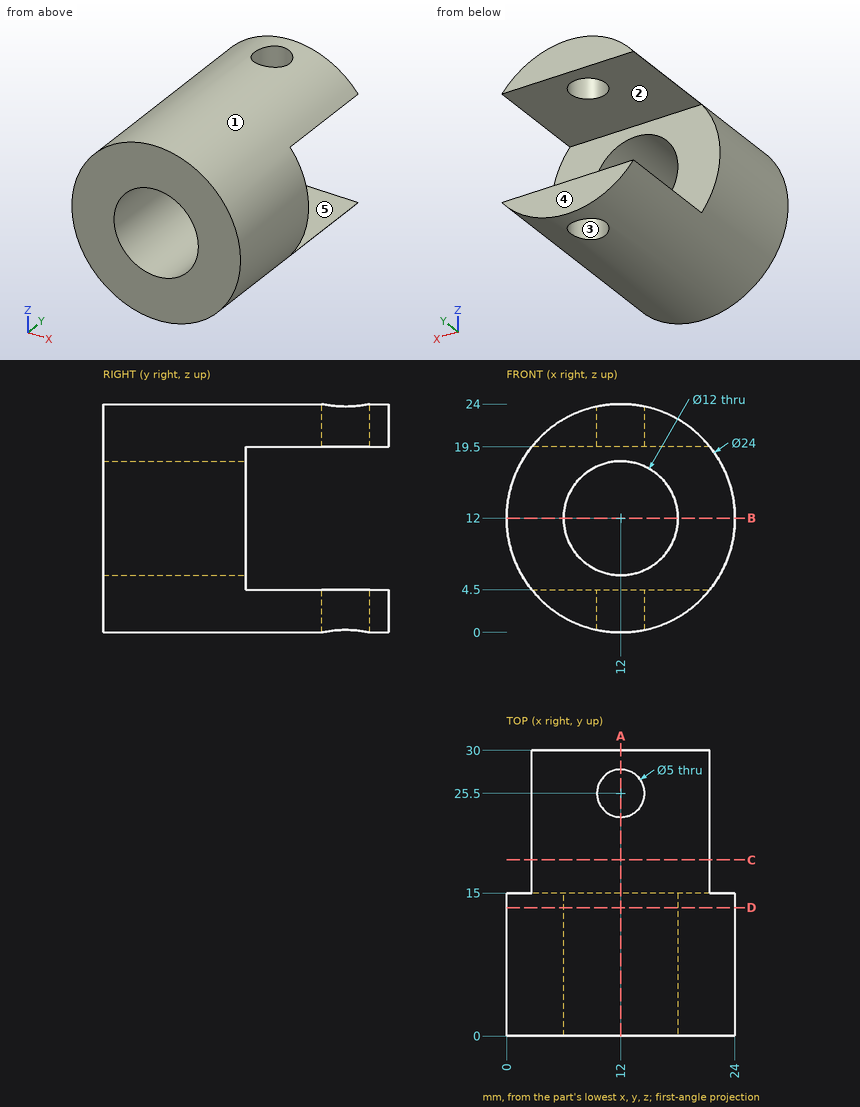
Verification items for this drawing (mm, ordinates from the low corner). A direction names the side the tool comes from. Round coordinates to 2 decimals unless told otherwise and drop trailing zeros. Write each loop counter-clockwise with the first axis right and the second up, starting at its lowest first coordinate (ties: lowest second). Pieces come first, ordered by that corner, then holes. Notation, with made-up numbers: (84, 89.5) - (118, 89.5) arc R25 ccw to (118, 116.5) - close; hole circle Ø6 at (-20, 75). An arc over 180 degrees is marked (long way). Answer as a JSON object with one key per item and string values. Group by question number.
Q1. Thickness scan on line 1 (Y direction, x = 12, z = 3.35); line 2 (Z direction, x = 12, y = 10); line 3 (Y direction, x = 3.5, z = 12.5). Record the ranges inside material, lowest first.
Q2. Mould release check, pull along Y, two halves, no side actions. Record for the marked faces 3, 4 and 5: released by +Y, released by -Y, zero draft, split by the parting line, or undercut.
Q3. Section check D-D, the plane y = 13.5. Enter the section's corners in (x, z), plus the area to 3 significant figures.
Q4. Tool access check on the marked faces 1 and 2. Record the directions out of +Z, -Z, +X, -X, +Y, -Y that give a thin tool (end or side, any length) a straight path to the whole face; none if there is none.
Q5. Section check C-C, the plane y = 18.5. Enter the section's corners in (x, z).
Q6. Section check B-B, the plane z = 12. Enter the section's corners in (x, y), plus the area to 3 significant figures.
Q7. Section check A-A, the plane x = 12. Enter the section's corners in (y, z).
Q8. Go/stop test with flat-tipped pins: pin 1 Ø4.5 at (x, z) = (13.5, 11) entering from +Y; pin 2 Ø4 at (x, y) = (20.5, 25.5) entering from -Z; pin 3 Ø5 at (x, y) = (17.5, 18.5) entering from +Z; pin 4 Ø1.5 at (x, y) = (10.5, 8.5) entering from +Z. Record where each tip stops, or that it passes through.
Found:
{
 "1": {"line 1": "y = 0 to 23, 28 to 30", "line 2": "z = 0 to 6, 18 to 24", "line 3": "y = 0 to 15"},
 "2": {"face 3": "undercut", "face 4": "released by +Y", "face 5": "zero draft"},
 "3": {"outline": "circle Ø24 at (12, 12); hole circle Ø12 at (12, 12)", "area": "339 mm^2"},
 "4": {"face 1": "+Y, -Y", "face 2": "+X, -X, +Y"},
 "5": {"outline": "(2.63, 4.5) arc R12 ccw to (21.37, 4.5) - close; (2.63, 19.5) - (21.37, 19.5) arc R12 ccw to start"},
 "6": {"outline": "(0, 0) - (6, 0) - (6, 15) - (0, 15) - close; (18, 0) - (24, 0) - (24, 15) - (18, 15) - close", "area": "180 mm^2"},
 "7": {"outline": "(0, 0) - (23, 0) - (23, 4.5) - (15, 4.5) - (15, 6) - (0, 6) - close; (0, 18) - (15, 18) - (15, 19.5) - (23, 19.5) - (23, 24) - (0, 24) - close; (28, 0) - (30, 0) - (30, 4.5) - (28, 4.5) - close; (28, 19.5) - (30, 19.5) - (30, 24) - (28, 24) - close"},
 "8": {"pin 1": "passes through", "pin 2": "stops at z = 1.91", "pin 3": "stops at z = 23.62", "pin 4": "stops at z = 23.98"}
}
